Verification items for the finished model (mm, model axes). Face numbers are marked on the shaded views. A direction names the side the tool comes from. Round coordinates to 2 decimals unless told otherwise and drop trailing zeros. Loops run counter-clockwise (first coordinate to the right, second up) from the corner with the lowest first, then second, coordinate; pieces in that order, holes last. Notation, with made-up numbers: (-35, 23) -> (-31, 23) arc R12 ccw to (-31, 39) -> close; hole circle Ø3 at (12, -33.5). An arc over 180 degrees is marked (long way). Use CSV: the item, a comma, the result in double quotes. Start each with the question number.
Autodesk Inventor part; units mm, degrees
ref_plane "YZ Plane" through (0, 0, 0) normal (1, 0, 0) x (0, 1, 0)
ref_plane "XZ Plane" through (0, 0, 0) normal (0, 1, 0) x (-1, 0, 0)
ref_plane "XY Plane" through (0, 0, 0) normal (0, 0, 1) x (1, 0, 0)
sketch "Sketch1" plane through (0, 0, 0) normal (0, 0, 1) x (1, 0, 0)
  line L0 (40, -65) -> (-40, -65)
  line L1 (-40, -65) -> (-40, 65)
  line L2 (-40, 65) -> (40, 65)
  line L3 (40, 65) -> (40, -65)
  line L4 (40, -65) -> (-40, 65) construction
  line L5 (-40, -65) -> (40, 65) construction
  point P0 (0, 0)
  dimension "d0" = 80
  dimension "d1" = 130
extrude "Extrusion1" add sketch "Sketch1" along normal blind 3
sketch "Sketch4" plane through (0, 0, 3) normal (0, 0, 1) x (1, 0, 0)
  line L0 (26.4795, -48.7045) -> (-26.4795, 48.7045) construction
  line L1 (-26.4795, -48.7045) -> (26.4795, 48.7045) construction
  circle A0 centre (-22.7965, 45.2755) radius 1.5
  circle A1 centre (23.0505, -45.2755) radius 1.5
  circle A2 centre (-22.7965, 45.2755) radius 4
  circle A3 centre (23.0505, -45.2755) radius 4
  point P0 (0, 0)
  dimension "d13" = 52.959
  dimension "d14" = 97.409
  dimension "d17" = 3
  dimension "d20" = 3
  dimension "d36" = 8
  dimension "d37" = 8
sketch "Sketch5" plane through (0, 0, 3) normal (0, 0, 1) x (1, 0, 0)
  line L0 (-40, 65) -> (-40, -65)
  line L1 (40, -65) -> (-40, -65)
  line L2 (-40, -65) -> (-40, 65)
  line L3 (40, 65) -> (40, -65)
  line L4 (36, -61) -> (-36, -61)
  line L5 (-36, -61) -> (-36, 61)
  line L6 (-36, 61) -> (36, 61)
  line L7 (36, 61) -> (36, -61)
  line L8 (40, 65) -> (-40, 65)
  line L9 (40, 65) -> (-40, 65)
  line L10 (-40, -65) -> (40, -65)
  point P0 (0, 0)
  dimension "d28" = 72
  dimension "d29" = 122
  dimension "d30" = 61
  dimension "d33" = 36
  dimension "d34" = 130
  dimension "d35" = 80
  dimension "d50" = 0
extrude "Extrusion4" add sketch "Sketch5" along normal blind 50
extrude "Extrusion5" add sketch "Sketch4" along normal blind 8
sketch "Sketch7" plane through (-22.7965, 45.2755, 11) normal (0, 0, 1) x (1, 0, 0)
  circle A0 centre (0, 0) radius 2.8
  point P0 (22.7965, -45.2755)
  dimension "d40" = 5.6
extrude "Extrusion6" cut sketch "Sketch7" against normal blind 3
sketch "Sketch8" plane through (23.0505, -45.2755, 11) normal (0, 0, 1) x (1, 0, 0)
  circle A0 centre (0, 0) radius 2.8
  point P0 (-23.0505, 45.2755)
  dimension "d43" = 5.6
extrude "Extrusion7" cut sketch "Sketch8" against normal blind 3
sketch "Sketch11" plane through (0, 0, 3) normal (0, 0, 1) x (1, 0, 0)
  circle A0 centre (-30, 55) radius 4
  circle A1 centre (30, 55) radius 4
  circle A2 centre (30, -55) radius 4
  circle A3 centre (-30, -55) radius 4
  line L0 (40, 65) -> (-40, 65)
  line L1 (-40, -65) -> (40, -65)
  circle A4 centre (-30, 55) radius 1.5
  circle A5 centre (30, 55) radius 1.5
  circle A6 centre (-30, -55) radius 1.5
  circle A7 centre (30, -55) radius 1.5
  point P0 (0, 0)
  dimension "d51" = 8
  dimension "d52" = 8
  dimension "d53" = 8
  dimension "d54" = 8
  dimension "d55" = 10
  dimension "d56" = 10
  dimension "d57" = 10
  dimension "d58" = 10
  dimension "d59" = 30
  dimension "d60" = 30
  dimension "d61" = 30
  dimension "d62" = 30
  dimension "d63" = 3
  dimension "d64" = 3
  dimension "d65" = 3
  dimension "d66" = 3
extrude "Extrusion8" add sketch "Sketch11" along normal blind 50
fillet "Fillet1" radius 5 8 edges at (40, -65, 26.5) (-40, -65, 26.5) (-40, 65, 26.5) (40, 65, 26.5) (-36, -61, 28) (36, -61, 28) (-36, 61, 28) (36, 61, 28)
properties part number "theMonarchPCBHolder"
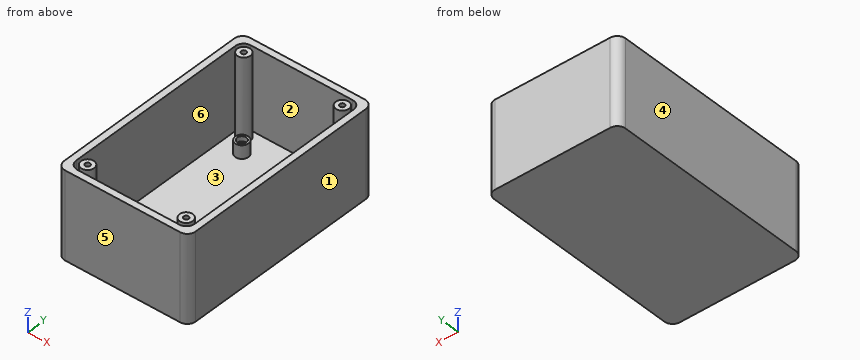
Q1. Cross-section at A-A (z = 19.5). State how many separate pieces and enclosed holes the cut face has, and give its area (3 significant figures).
Q2. Release check for a two-part mould opening along Y. For the marked faces 3, 4, 5 and 6 record: +Y half, -Y half, draft (parallel to the pull), parting line (faces both ways), or undercut.
Q3. Depth check by flat-ended pin: pin 1 Ø0.9 at (x, y) = (-30, -55.5) entering from +Z; pin 2 Ø6 at (x, y) = (-23, 45.5) entering from +Z; pin 3 Ø1.7 at (x, y) = (23, -44) entering from +Z. Enter the tip coordinate at first touch or a pass-through.
Q4. Tool access check on the marked faces 1 and 2. Record the directions out of +Z, -Z, +X, -X, +Y, -Y that give a thin tool (end or side, any length) a straight path to the whole face; none if there is none.
Q5. Cross-section at B-B (y = 15). Record the boundary of the cut face in (x, z).
Q6. Thickness scan on L1, parallel to Y at x = 30, z = 26; L2, parallel to X at y = 2, z = 23; L3, parallel to Y at x = 11, z = 44. Record the ranges inside material, lowest first. Write a range as from..to.
Q7. Cross-section at C-C (x = -2.5). Record the boundary of the cut face in (y, z).
Answer list:
1,separate pieces,"5"
1,enclosed holes,"5"
1,area,"1,790 mm2"
2,face 3,"undercut"
2,face 4,"draft"
2,face 5,"-Y half"
2,face 6,"undercut"
3,pin 1,"stops at z = 3"
3,pin 2,"stops at z = 11"
3,pin 3,"stops at z = 8"
4,face 1,"+Z, -Z, +X, +Y, -Y"
4,face 2,"+Z"
5,outline,"(-40, 0) -> (40, 0) -> (40, 53) -> (36, 53) -> (36, 3) -> (-36, 3) -> (-36, 53) -> (-40, 53) -> close"
6,L1,"y = -65..-61, -59..-56.5, -53.5..-51, 51..53.5, 56.5..59, 61..65"
6,L2,"x = -40..-36, 36..40"
6,L3,"y = -65..-61, 61..65"
7,outline,"(-65, 0) -> (65, 0) -> (65, 53) -> (61, 53) -> (61, 3) -> (-61, 3) -> (-61, 53) -> (-65, 53) -> close"
